from build123d import *

# Parameters (mm, degrees)
BOSS_EXTRU_1_DEPTH      = 77.05
ESQUISSE3_W             = 10
ESQUISSE3_H             = 6.35
BOSS_EXTRU_2_DEPTH      = 1
ESQUISSE5_W             = 1.539298861
ESQUISSE5_H             = 1.197636308
ESQUISSE5_W_2           = 1.565261684
ENL_V_MAT_EXTRU_1_DEPTH = 1
ESQUISSE6_W             = 73.632054576
ESQUISSE6_H             = 17.392646246
ENL_V_MAT_EXTRU_2_DEPTH = 14
ESQUISSE7_W             = 71.72564692
ESQUISSE7_H             = 6.995918618
ENL_V_MAT_EXTRU_3_DEPTH = 16
ESQUISSE8_W             = 12
ESQUISSE8_H             = 8.25967539
ESQUISSE8_W_2           = 17.68111001
ENL_V_MAT_EXTRU_4_DEPTH = 23
CONG_1_R                = 10


with BuildPart() as part:
    # Esquisse1 → Boss.-Extru.1 (new body)
    with BuildSketch(Plane(origin=(0, 0, 0), x_dir=(0, 0, -1), z_dir=(1, 0, 0))):
        Polygon((-10.5, 10.9), (-9.1, 14.9), (9.1, 14.9), (10.5, 10.9), (10.5, 0), (-10.5, 0), align=None)
    extrude(amount=BOSS_EXTRU_1_DEPTH)

    # Esquisse3 → Boss.-Extru.2 (add)
    with BuildSketch(Plane.XZ):
        Rectangle(ESQUISSE3_W, ESQUISSE3_H)
        with Locations((77.05, 0)):
            Rectangle(ESQUISSE3_W, ESQUISSE3_H)
    extrude(amount=-BOSS_EXTRU_2_DEPTH)

    # Esquisse5 → Enlèv. mat.-Extru.1 (cut)
    with BuildSketch(Plane.XZ):
        with Locations((-3.397480153, 0)):
            Rectangle(ESQUISSE5_W, ESQUISSE5_H)
        with Locations((80.22152685, 0)):
            Rectangle(ESQUISSE5_W_2, ESQUISSE5_H)
    extrude(amount=-ENL_V_MAT_EXTRU_1_DEPTH, mode=Mode.SUBTRACT)

    # Esquisse6 → Enlèv. mat.-Extru.2 (cut)
    with BuildSketch(Plane(origin=(0, 14.9, 0), x_dir=(1, 0, 0), z_dir=(0, 1, 0))):
        with Locations((38.525, 0)):
            Rectangle(ESQUISSE6_W, ESQUISSE6_H)
    extrude(amount=-ENL_V_MAT_EXTRU_2_DEPTH, mode=Mode.SUBTRACT)

    # Esquisse7 → Enlèv. mat.-Extru.3 (cut)
    with BuildSketch(Plane(origin=(0, 14.9, 0), x_dir=(1, 0, 0), z_dir=(0, 1, 0))):
        with Locations((38.525, 0)):
            Rectangle(ESQUISSE7_W, ESQUISSE7_H)
    extrude(amount=-ENL_V_MAT_EXTRU_3_DEPTH, mode=Mode.SUBTRACT)

    # Esquisse8 → Enlèv. mat.-Extru.4 (cut)
    with BuildSketch(Plane.XY.offset(10.5)):
        with Locations((8.5, 10.770162305)):
            Rectangle(ESQUISSE8_W, ESQUISSE8_H)
        with Locations((38.340555005, 10.770162305)):
            Rectangle(ESQUISSE8_W_2, ESQUISSE8_H)
        with Locations((68.18111001, 10.770162305)):
            Rectangle(ESQUISSE8_W, ESQUISSE8_H)
    extrude(amount=-ENL_V_MAT_EXTRU_4_DEPTH, mode=Mode.SUBTRACT)

    # Congé1
    cong_1_edges = [part.edges().sort_by_distance(p)[0] for p in [
        (75.615555005, 10.9, 10.5),
        (75.615555005, 10.9, -10.5),
        (1.25, 10.9, 10.5),
        (1.25, 10.9, -10.5),
        (22, 10.9, 10.5),
        (22, 10.9, -10.5),
        (54.68111001, 10.9, 10.5),
        (54.68111001, 10.9, -10.5),
    ]]
    fillet(cong_1_edges, radius=CONG_1_R)


solid = part.part
Can you work these out from the model? Positions are in its coordinate system, mm. A direction names the side the tool comes from. Coordinates: 2 decimals unless noted, no trailing zeros. Write each loop counter-clockwise with the first axis right and the second up, starting at its lowest first coordinate (ties: lowest second). Pieces come first, ordered by that corner, then holes. Notation, with made-up numbers: M -5.5,-15 L 33.5,-15 A19 cw 33.5,-3 Z; hole C 75,13 d11. An arc over 180 degrees is marked long. Use one line per item in the form item = value.
Q1. For faces 1 (the flat face through (-2, 1, 0)), 2 (the flat face through (38, 5, -8.696)), 3 (the flat face through (47.181, 10, -9)), which set-ups out of +Z, -Z, +X, -X, +Y, -Y let a thin tool reach every point of the face, with its end or its side?
Model answer:
face_1 = +Z, -Z, -X, +Y
face_2 = +Y
face_3 = +Z, -Z, +Y
Q2. For P1, Ø1.1, axis at x = -3, y = 0.5, coming from the -Z side (3 decimals); P2, Ø1.1, axis at x = 80.5, y = 0.5, coming from the +Z side (3 decimals); P3, Ø0.9, axis at y = 9, z = 9, coming from the -X side, each with a flat end and sliding along its axis, tell me the tip position at first contact or that it passes through.
Model answer:
P1 = -3.175
P2 = 3.175
P3 = 0
Q3. If we section it at D-D (y = 3.25): Write out the boundary of the cut face in (x, z).
Model answer:
outline = M 0,-10.5 L 77.05,-10.5 L 77.05,10.5 L 0,10.5 Z; hole M 1.71,-8.7 L 75.34,-8.7 L 75.34,8.7 L 1.71,8.7 Z
Q4. If we section it at B-B (y = 13.5): State how many separate pieces and enclosed holes the cut face has, then the cut area to 3 significant figures.
Model answer:
separate_pieces = 6
enclosed_holes = 0
area = 123 mm^2
Q5. I need wall thicknesses on line 1 along X through (y, z) = (6.75, -6); line 2 along Z through (x, y) = (6, 6.25); line 3 along Y through (x, z) = (67.5, 5). Which ranges of each line are inside material? Lowest first, please. Write a range as from..to.
Model answer:
line_1 = 0..1.71, 75.34..77.05
line_2 = -10.5..-8.7, 8.7..10.5
line_3 = 0..0.9
Q6. We'd pull the mould along X, two halves only. Please class faces 4 (the cylindrical face through (54.786, 10.853, 10.363)), 5 (the flat face through (62.181, 10, -9)): +X half, -X half, draft (parallel to the pull), parting line (faces both ways), or undercut.
Model answer:
face_4 = draft
face_5 = undercut
Q7. If we section it at C-C (z = 7.5): Write out the boundary of the cut face in (x, y), then the cut area to 3 significant figures.
Model answer:
outline = M 0,0 L 77.05,0 L 77.05,14.9 L 75.34,14.9 L 75.34,0.9 L 1.71,0.9 L 1.71,14.9 L 0,14.9 Z
area = 117 mm^2
Q8. If we section it at A-A (x = 27.5): Write out the boundary of the cut face in (y, z).
Model answer:
outline = M 0,-10.5 L 9.2,-10.5 A10 ccw 12.5,-9.94 L 14.9,-9.1 L 14.9,-8.7 L 0.9,-8.7 L 0.9,-3.5 L 0,-3.5 Z; M 0,3.5 L 0.9,3.5 L 0.9,8.7 L 14.9,8.7 L 14.9,9.1 L 12.5,9.94 A10 ccw 9.2,10.5 L 0,10.5 Z
